Could you check a few things on this model? Use its own coordinates, in mm. A direction names the side the tool comes from. Round coordinates to 2 decimals unless told otherwise and drop trailing zeros. Loops run counter-clockwise (first coordinate to the right, second up) from the corner with the lowest first, then second, coordinate; pieces in that order, holes last. Notation, with made-up numbers: (-39, 61) - (-6, 61) arc R16 ccw to (-6, 74) - close; hole circle Ø1 at (87, -9.5). An arc over 180 degrees is marked (long way). Put each result on its own line as item: value. Start each with the question number.
from build123d import *

# Parameters (mm, degrees)
F0_R     = 75
F1_DEPTH = 10
F2_R     = 1.775
F2_R_2   = 1.762154
F3_DEPTH = 25
F4_W     = 5
F4_H     = 30
F5_DEPTH = 25


with BuildPart() as f1:
    # F0 (on Top) → F1 (new body)
    with BuildSketch(Plane.XY):
        Circle(F0_R)
    extrude(amount=F1_DEPTH)

    # F2 (on face) → F3 (cut)
    with BuildSketch(Plane.XY.offset(10)):
        with Locations((-35, 35)):
            Circle(F2_R)
        with Locations((-25, 25)):
            Circle(F2_R_2)
        with Locations((25, 25)):
            Circle(F2_R)
        with Locations((35, 35)):
            Circle(F2_R)
        with Locations((25, -25)):
            Circle(F2_R)
        with Locations((35, -35)):
            Circle(F2_R)
        with Locations((-25, -25)):
            Circle(F2_R)
        with Locations((-35, -35)):
            Circle(F2_R)
    extrude(amount=-F3_DEPTH, mode=Mode.SUBTRACT)

    # F4 (on face) → F5 (cut)
    with BuildSketch(Plane.XY.offset(10)):
        with Locations((-42.5, 0)):
            Rectangle(F4_W, F4_H)
        with Locations((42.5, 0)):
            Rectangle(F4_W, F4_H)
    extrude(amount=-F5_DEPTH, mode=Mode.SUBTRACT)


solid = f1.part
Item 1: Suppose I cut it at C-C, the plane x = 25. List the corners of the cut face in (y, z) for me (3 decimals), then the cut area to 3 significant figures.
Item 2: Will these pins go through, and if not, where does the flat tip stop? P1, Ø5.5, axis at x = -25, y = 25, coming from the -Z side; P2, Ø4, axis at x = -43.5, z = 6, coming from the -Y side; P3, Ø3, axis at y = -5.5, z = 3.5, coming from the -X side; P4, Ø3, axis at y = 46.5, z = 5, coming from the +X side.
Item 3: Suppose I cut it at A-A, the plane y = 0. List the corners of the cut face in (x, z) for me, then the cut area to 3 significant figures.
Item 4: I need wall thicknesses on line 1 (X direction, y = 26.5, z = 7.5); line 2 (Y direction, x = -35, z = 3.75) (1 decimal); line 3 (Y direction, x = -25, z = 4.5) (3 decimals). Which ranges of each line are inside material? Lowest first, please. Write a range as from..to.
Item 5: Thinking about a two-plate mould opening in X: for faces 1 (the face through (-45, 0, 5)), 2 (the face through (36.693, -34.467, 5.07)), 3 (the face through (-9.764, 74.362, 4.93)), 4 (the face through (-1, 1, 10)), which applies, released by +X, released by -X, zero draft, split by the parting line, or undercut?
Item 6: On a 3-axis mill with a long thin cutter (end or side, diameter ignored), from which of +Z, -Z, +X, -X, +Y, -Y can I reach the whole of each face in a straight line? I mean faces 5 (the face through (-1, 1, 0)), 6 (the face through (42, -15, 5)). Say none if no direction works.
Item 7: Suppose I cut it at B-B, the plane z = 1.75. Count the separate pieces of the cut face and the enclosed holes in it, then the cut area to 3 significant figures.
Item 8: Suppose I cut it at D-D, the plane y = 47. List the corners of the cut face in (x, z) for me.
Numbers:
1. outline: (-70.711, 0) - (-26.775, 0) - (-26.775, 10) - (-70.711, 10) - close; (-23.225, 0) - (23.225, 0) - (23.225, 10) - (-23.225, 10) - close; (26.775, 0) - (70.711, 0) - (70.711, 10) - (26.775, 10) - close
1. area: 1,340 mm^2
2. P1: z = 0
2. P2: y = -62.47
2. P3: x = -74.89
2. P4: x = 60
3. outline: (-75, 0) - (-45, 0) - (-45, 10) - (-75, 10) - close; (-40, 0) - (40, 0) - (40, 10) - (-40, 10) - close; (45, 0) - (75, 0) - (75, 10) - (45, 10) - close
3. area: 1,400 mm^2
4. line 1: -70.16..-25.92, -24.08..24.05, 25.95..70.16
4. line 2: -66.3..-36.8, -33.2..33.2, 36.8..66.3
4. line 3: -70.711..-26.775, -23.225..23.238, 26.762..70.711
5. face 1: undercut
5. face 2: undercut
5. face 3: split by the parting line
5. face 4: zero draft
6. face 5: -Z, +X, -X, +Y, -Y
6. face 6: +Z, -Z
7. separate pieces: 1
7. enclosed holes: 10
7. area: 17,300 mm^2
8. outline: (-58.45, 0) - (58.45, 0) - (58.45, 10) - (-58.45, 10) - close
